```python
from build123d import *

# Parameters (mm, degrees)
F1_DEPTH    = 2.3
F2_R        = 2.25
F3_DEPTH    = 25
F4_T1_DEPTH = 49.9198715888


# Not quite as in the source:
# - a fillet or chamfer that OpenCascade refuses, or shapes differently, is made with other operations: its cross-section is extruded or revolved along the edge and cut away or added


with BuildPart() as f1:
    # F0 (on Top) → F1 (new body, symmetric)
    with BuildSketch(Plane.XY):
        Polygon((12.5, 22.5), (-12.5, 22.5), (-12.5, 16.1530176364), (-8.5, 16.1530176364), (-8.5, 11.1530176364), (-12.5, 11.1530176364), (-12.5, -11.1530176364), (-8.5, -11.1530176364), (-8.5, -16.1530176364), (-12.5, -16.1530176364), (-12.5, -22.5), (12.5, -22.5), (12.5, -16.1530176364), (8.5, -16.1530176364), (8.5, -11.1530176364), (12.5, -11.1530176364), (12.5, 11.1530176364), (8.5, 11.1530176364), (8.5, 16.1530176364), (12.5, 16.1530176364), align=None)
    extrude(amount=F1_DEPTH, both=True)

    # F2 (on face) → F3 (cut)
    with BuildSketch(Plane.YZ.offset(8.5)):
        with Locations((-13.6288348585, 0.6045123446)):
            Circle(F2_R)
        with Locations((13.6288348585, 0.6045123446)):
            Circle(F2_R)
    extrude(amount=-F3_DEPTH, mode=Mode.SUBTRACT)

    # F4: fillet of radius 5 on 2 edges, made by hand

    # F4_s2 → F4_t1 (cut)
    with BuildSketch(Plane.YZ.offset(-24.9599357944)):
        with BuildLine():
            ThreePointArc((-22.5, 2.3), (-20.9071906738, -0.9742346142), (-17.5160256822, -2.3))
            Line((-17.5160256822, -2.3), (-22.5, -2.3))
            Line((-22.5, -2.3), (-22.5, 2.3))
        make_face()
        with BuildLine():
            ThreePointArc((22.5, 2.3), (20.9071906738, -0.9742346142), (17.5160256822, -2.3))
            Line((17.5160256822, -2.3), (22.5, -2.3))
            Line((22.5, -2.3), (22.5, 2.3))
        make_face()
    extrude(amount=F4_T1_DEPTH, mode=Mode.SUBTRACT)


solid = f1.part
```
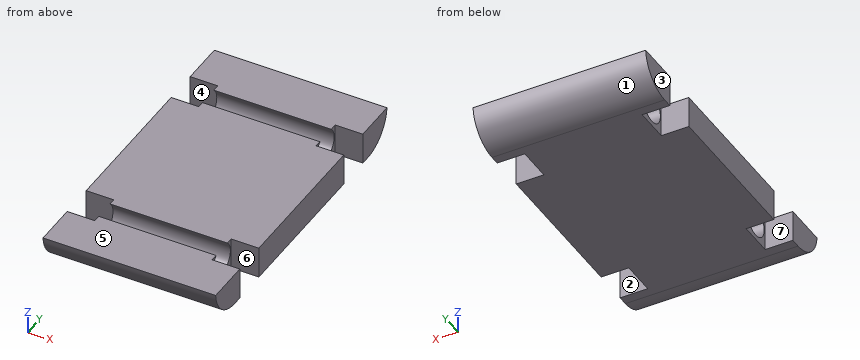
Part model, mm, in its own coordinate system. Face numbers are marked on the shaded views. A direction names the side the tool comes from. Round coordinates to 2 decimals unless told otherwise and drop trailing zeros. Loops run counter-clockwise (first coordinate to the right, second up) from the corner with the lowest first, then second, coordinate; pieces in that order, holes last.
1. Drill centre lines: line 1 along Y through (x, z) = (1.25, 1.55); line 2 along Y through (x, z) = (2.5, -1.4); line 3 along Z through (x, y) = (-5, 13.5). Where is each one in solid material? Low to high.
Solutions:
line 1: y = -22.38 to -15.67, -11.59 to 11.59, 15.67 to 22.38
line 2: y = -20.38 to -14.65, -12.61 to 12.61, 14.65 to 20.38
line 3: z = -2.3 to -1.64
2. Slice it at C-C (z = 1.8). Give the cut face in (x, y), and give its area (3 significant figures).
Solutions:
outline: (-12.5, -22.43) - (12.5, -22.43) - (12.5, -16.15) - (8.5, -16.15) - (8.5, -15.53) - (-8.5, -15.53) - (-8.5, -16.15) - (-12.5, -16.15) - close; (-12.5, -11.15) - (-8.5, -11.15) - (-8.5, -11.72) - (8.5, -11.72) - (8.5, -11.15) - (12.5, -11.15) - (12.5, 11.15) - (8.5, 11.15) - (8.5, 11.72) - (-8.5, 11.72) - (-8.5, 11.15) - (-12.5, 11.15) - close; (-12.5, 16.15) - (-8.5, 16.15) - (-8.5, 15.53) - (8.5, 15.53) - (8.5, 16.15) - (12.5, 16.15) - (12.5, 22.43) - (-12.5, 22.43) - close
area: 912 mm2
3. Slice it at A-A (x = -9.25). Give the cut face in (y, z).
Solutions:
outline: (-22.5, 2.3) arc R5 ccw to (-17.52, -2.3) - (-16.15, -2.3) - (-16.15, 2.3) - close; (-11.15, -2.3) - (11.15, -2.3) - (11.15, 2.3) - (-11.15, 2.3) - close; (16.15, -2.3) - (17.52, -2.3) arc R5 ccw to (22.5, 2.3) - (16.15, 2.3) - close
4. 3-axis set-ups, long thin cutter, end or side, ignore diameter. For the marked faces 5, 6 and 7: which of +Z, -Z, +X, -X, +Y, -Y reach the whole face in a straight line?
Solutions:
face 5: +Z, +X, -X, +Y, -Y
face 6: +Z, -Z, +X
face 7: +Z, -Z, -X
5. Slice it at D-D (z = -0.6). Give the cut face in (x, y).
Solutions:
outline: (-12.5, -21.27) - (12.5, -21.27) - (12.5, -16.15) - (8.5, -16.15) - (8.5, -15.53) - (-8.5, -15.53) - (-8.5, -16.15) - (-12.5, -16.15) - close; (-12.5, -11.15) - (-8.5, -11.15) - (-8.5, -11.73) - (8.5, -11.73) - (8.5, -11.15) - (12.5, -11.15) - (12.5, 11.15) - (8.5, 11.15) - (8.5, 11.73) - (-8.5, 11.73) - (-8.5, 11.15) - (-12.5, 11.15) - close; (-12.5, 16.15) - (-8.5, 16.15) - (-8.5, 15.53) - (8.5, 15.53) - (8.5, 16.15) - (12.5, 16.15) - (12.5, 21.27) - (-12.5, 21.27) - close
6. Two-plate mould, pull along Y, no slides. Class the marked faces 1, 2, 3 and 4: pulls with the +Y half, pulls with the -Y half, needs draft (parallel to the pull), parting line crosses it, or undercut.
Solutions:
face 1: pulls with the +Y half
face 2: undercut
face 3: needs draft
face 4: undercut
7. Slice it at B-B (x = 6.75). Give the cut face in (y, z).
Solutions:
outline: (-22.5, 2.3) arc R5 ccw to (-17.52, -2.3) - (17.52, -2.3) arc R5 ccw to (22.5, 2.3) - (15.11, 2.3) arc R2.25 cw (long way) to (12.15, 2.3) - (-12.15, 2.3) arc R2.25 cw (long way) to (-15.11, 2.3) - close
8. Flat gauge pins, fed straight in: pin 1 (1.5 mm diameter, centred on x = -9, z = 1.5, fed in from -Y); pin 2 (1.2 mm diameter, centred on x = -11, z = 0.5, fed in from +Y); pin 3 (2 mm diameter, centred on x = -10.5, z = 0, fed in from -Y). Where does each tip first touch, or does it go through?
Solutions:
pin 1: stops at y = -22.5
pin 2: stops at y = 22.25
pin 3: stops at y = -22.22
